Design review of the part built by this model. Coordinates are the model's own, in mm. Give positions to 0.01 mm unless a question says otherwise; leave off trailing zeros. Loops run counter-clockwise (first coordinate to the right, second up) from the corner with the lowest first, then second, coordinate; pieces in that order, holes last. Notation, with made-up numbers: (1.25, 35) - (33.25, 35) arc R18 ccw to (33.25, 70) - close; hole circle Ø3 at (-7.75, 73.5). An arc over 180 degrees is marked (long way). Write each question's results on one line, items separated by ' | '.
from build123d import *

# Parameters (mm, degrees)
SKETCH1_W           = 120
SKETCH1_H           = 120
BOSS_EXTRUDE1_DEPTH = 3
SKETCH4_R           = 5
CUT_EXTRUDE2_DEPTH  = 3
SKETCH7_R           = 1.5
CUT_EXTRUDE3_DEPTH  = 3


with BuildPart() as part:
    # Sketch1 → Boss-Extrude1 (new body)
    with BuildSketch(Plane(origin=(0, 0, 0), x_dir=(1, 0, 0), z_dir=(0, 1, 0))):
        Rectangle(SKETCH1_W, SKETCH1_H)
    extrude(amount=BOSS_EXTRUDE1_DEPTH)

    # Sketch4 → Cut-Extrude2 (cut)
    with BuildSketch(Plane(origin=(0, 0, 0), x_dir=(1, 0, 0), z_dir=(0, 1, 0))):
        with Locations((-22.5, 0)):
            Circle(SKETCH4_R)
        with Locations((22.5, 0)):
            Circle(SKETCH4_R)
    extrude(amount=CUT_EXTRUDE2_DEPTH, mode=Mode.SUBTRACT)

    # Sketch7 → Cut-Extrude3 (cut)
    with BuildSketch(Plane(origin=(0, 0, 0), x_dir=(1, 0, 0), z_dir=(0, 1, 0))):
        with Locations((-53, 53)):
            Circle(SKETCH7_R)
        with Locations((53, 53)):
            Circle(SKETCH7_R)
        with Locations((-53, -53)):
            Circle(SKETCH7_R)
        with Locations((53, -53)):
            Circle(SKETCH7_R)
    extrude(amount=CUT_EXTRUDE3_DEPTH, mode=Mode.SUBTRACT)


solid = part.part
(1) Take a section at C-C on x = 53. Give the boundary of the cut face in (y, z), plus the area to 3 significant figures.
Answers below:
outline: (0, -60) - (3, -60) - (3, -54.5) - (0, -54.5) - close; (0, -51.5) - (3, -51.5) - (3, 51.5) - (0, 51.5) - close; (0, 54.5) - (3, 54.5) - (3, 60) - (0, 60) - close | area: 342 mm2
(2) Take a section at A-A on z = -53. Give the boundary of the cut face in (x, y).
Answers below:
outline: (-60, 0) - (-54.5, 0) - (-54.5, 3) - (-60, 3) - close; (-51.5, 0) - (51.5, 0) - (51.5, 3) - (-51.5, 3) - close; (54.5, 0) - (60, 0) - (60, 3) - (54.5, 3) - close
(3) Take a section at B-B on x = -22.5. Give the boundary of the cut face in (y, z), plus the area to 3 significant figures.
Answers below:
outline: (0, -60) - (3, -60) - (3, -5) - (0, -5) - close; (0, 5) - (3, 5) - (3, 60) - (0, 60) - close | area: 330 mm2
(4) Take a section at D-D on x = 23. Give the boundary of the cut face in (y, z), plus the area to 3 significant figures.
Answers below:
outline: (0, -60) - (3, -60) - (3, -4.97) - (0, -4.97) - close; (0, 4.97) - (3, 4.97) - (3, 60) - (0, 60) - close | area: 330 mm2
(5) Wall thickness on line 1 along Z through (x, y) = (53, 1.95); line 2 along X through (y, z) = (2.15, 0): over which ranges is each line inside the solid? List them lowest first. Write a range as from..to.
Answers below:
line 1: -60..-54.5, -51.5..51.5, 54.5..60 | line 2: -60..-27.5, -17.5..17.5, 27.5..60
(6) Insertion check: P1, Ø2.5, axis at x = 53, z = 53, coming from the -Y side. The pin has a flat end and moves straight along its axis. Give the tip position at first contact, or say it passes through.
Answers below:
P1: through
(7) Draft analysis for pull direction X (two halves, no side actions). For faces 1 (the flat face through (-60, 1, 1)), 2 (the cylindrical face through (51.8, 1.5, 53.9)), 3 (the flat face through (60, 1, 1)), 4 (the flat face through (-1, 3, -1)), state which applies: pulls with the +X half, pulls with the -X half, needs draft (parallel to the pull), parting line crosses it, or undercut.
Answers below:
face 1: pulls with the -X half | face 2: undercut | face 3: pulls with the +X half | face 4: needs draft
